```python
from build123d import *

# Parameters (mm, degrees)
SKETCH1_W                        = 20
SKETCH1_H                        = 20
BOSS_EXTRUDE1_DEPTH              = 30
F_3_0MM_DOWEL_HOLE1_D            = 3
F_3_0MM_DOWEL_HOLE1_DEPTH        = 20
F_3_0MM_DOWEL_HOLE1_CSINK_D      = 3.05
F_3_0MM_DOWEL_HOLE1_CSINK_ANGLE  = 90
F_3_0MM_DOWEL_HOLE1_TIP          = 0.901290929
F_3_0MM_DOWEL_HOLE2_D            = 3
F_3_0MM_DOWEL_HOLE2_DEPTH        = 12
F_3_0MM_DOWEL_HOLE2_CSINK_D      = 3.05
F_3_0MM_DOWEL_HOLE2_CSINK_ANGLE  = 90
F_3_0MM_DOWEL_HOLE2_TIP          = 0.901290929
F_3_0MM_DOWEL_HOLE3_D            = 3
F_3_0MM_DOWEL_HOLE3_DEPTH        = 20
F_3_0MM_DOWEL_HOLE3_CSINK_D      = 3.05
F_3_0MM_DOWEL_HOLE3_CSINK_ANGLE  = 90
F_3_0MM_DOWEL_HOLE3_TIP          = 0.901290929
F_10_0MM_DOWEL_HOLE1_D           = 9
F_10_0MM_DOWEL_HOLE1_DEPTH       = 17
F_10_0MM_DOWEL_HOLE1_CSINK_D     = 10.05
F_10_0MM_DOWEL_HOLE1_CSINK_ANGLE = 90
F_10_0MM_DOWEL_HOLE1_TIP         = 2.703872786


with BuildPart() as part:
    # Sketch1 → Boss-Extrude1 (new body)
    with BuildSketch(Plane(origin=(0, 0, 0), x_dir=(1, 0, 0), z_dir=(0, 1, 0))):
        with Locations((10, -8.099538279)):
            Rectangle(SKETCH1_W, SKETCH1_H)
    extrude(amount=BOSS_EXTRUDE1_DEPTH)

    # Ø3.0mm Dowel Hole1
    with Locations(Plane(origin=(0, 0, -1.900461721), x_dir=(-1, 0, 0), z_dir=(0, 0, -1))):
        with Locations((-16, 20)):
            CounterSinkHole(F_3_0MM_DOWEL_HOLE1_D / 2, F_3_0MM_DOWEL_HOLE1_CSINK_D / 2, depth=F_3_0MM_DOWEL_HOLE1_DEPTH, counter_sink_angle=F_3_0MM_DOWEL_HOLE1_CSINK_ANGLE)
            with Locations((0, 0, -(F_3_0MM_DOWEL_HOLE1_DEPTH + F_3_0MM_DOWEL_HOLE1_TIP / 2))):  # 118° drill point
                Cone(0, F_3_0MM_DOWEL_HOLE1_D / 2, F_3_0MM_DOWEL_HOLE1_TIP, mode=Mode.SUBTRACT)

    # Ø3.0mm Dowel Hole2
    with Locations(Plane.ZY):
        with Locations((10.099538279, 20)):
            CounterSinkHole(F_3_0MM_DOWEL_HOLE2_D / 2, F_3_0MM_DOWEL_HOLE2_CSINK_D / 2, depth=F_3_0MM_DOWEL_HOLE2_DEPTH, counter_sink_angle=F_3_0MM_DOWEL_HOLE2_CSINK_ANGLE)
            with Locations((0, 0, -(F_3_0MM_DOWEL_HOLE2_DEPTH + F_3_0MM_DOWEL_HOLE2_TIP / 2))):  # 118° drill point
                Cone(0, F_3_0MM_DOWEL_HOLE2_D / 2, F_3_0MM_DOWEL_HOLE2_TIP, mode=Mode.SUBTRACT)

    # Ø3.0mm Dowel Hole3
    with Locations(Plane(origin=(0, 30, 0), x_dir=(1, 0, 0), z_dir=(0, 1, 0))):
        with Locations((8, -4.099538279)):
            CounterSinkHole(F_3_0MM_DOWEL_HOLE3_D / 2, F_3_0MM_DOWEL_HOLE3_CSINK_D / 2, depth=F_3_0MM_DOWEL_HOLE3_DEPTH, counter_sink_angle=F_3_0MM_DOWEL_HOLE3_CSINK_ANGLE)
            with Locations((0, 0, -(F_3_0MM_DOWEL_HOLE3_DEPTH + F_3_0MM_DOWEL_HOLE3_TIP / 2))):  # 118° drill point
                Cone(0, F_3_0MM_DOWEL_HOLE3_D / 2, F_3_0MM_DOWEL_HOLE3_TIP, mode=Mode.SUBTRACT)

    # Ø10.0mm Dowel Hole1
    with Locations(Plane(origin=(20, 0, 0), x_dir=(0, 0, -1), z_dir=(1, 0, 0))):
        with Locations((-6.099538279, 8)):
            CounterSinkHole(F_10_0MM_DOWEL_HOLE1_D / 2, F_10_0MM_DOWEL_HOLE1_CSINK_D / 2, depth=F_10_0MM_DOWEL_HOLE1_DEPTH, counter_sink_angle=F_10_0MM_DOWEL_HOLE1_CSINK_ANGLE)
            with Locations((0, 0, -(F_10_0MM_DOWEL_HOLE1_DEPTH + F_10_0MM_DOWEL_HOLE1_TIP / 2))):  # 118° drill point
                Cone(0, F_10_0MM_DOWEL_HOLE1_D / 2, F_10_0MM_DOWEL_HOLE1_TIP, mode=Mode.SUBTRACT)


solid = part.part
```
The listing builds one solid part. Answer for the finished solid, in the listing's coordinates (mm). A direction names the side the tool comes from. Round coordinates to 2 decimals unless told otherwise and drop trailing zeros. Write each loop counter-clockwise with the first axis right and the second up, starting at its lowest first coordinate (ties: lowest second). Pieces come first, ordered by that corner, then holes. Notation, with made-up numbers: (11.5, -38) -> (38.5, -38) arc R19 ccw to (38.5, -27) -> close; hole circle Ø3 at (26, 64). An arc over 180 degrees is marked (long way). Use CSV: the item, a comma, the result in double quotes. Start each with the question number.
(1) Section B-B on x = 13.5 is taken. Give the vertices of the cut face in (y, z).
(2) The mould has two halves that part along Z. Classify faces 5 (the face through (14.89, 21.01, 8.25)), 6 (the face through (0.766, 8.775, 6.201)), 7 (the face through (10, 15, -1.9)): released by +Z, released by -Z, zero draft, split by the parting line, or undercut.
(3) Section D-D on y = 25.75 is taken. Give the vertices of the cut face in (x, z), then the cut area to 3 significant figures.
(4) Section A-A on x = 16 is taken. Give the vertices of the cut face in (y, z) (3 decimals).
(5) Consider L1, parallel to Z at x = 8, y = 19.25; L2, parallel to Y at x = 11.25, z = 9.75; L3, parallel to X at y = 20, z = 4.75. Determine where each line is inside the solid, lowest interval first. Write a range as from..to.
(6) Section C-C on x = 10 is taken. Give the vertices of the cut face in (y, z).
(7) Which of the six approach directions +Z, -Z, +X, -X, +Y, -Y give full straight-line access (tool end or side, diameter ignored) to faces 1 (the face through (11.12, 6.28, 10.26)), 2 (the face through (8.195, 20.268, 2.612)), 3 (the face through (6.096, 21.265, 9.293)), 4 (the face through (20, 15, 8))?
A:
1,outline,"(0, -1.9) -> (30, -1.9) -> (30, 18.1) -> (0, 18.1) -> close; hole circle Ø9 at (8, 6.1)"
2,face 5,"zero draft"
2,face 6,"undercut"
2,face 7,"released by -Z"
3,outline,"(0, -1.9) -> (20, -1.9) -> (20, 18.1) -> (0, 18.1) -> close; hole circle Ø3 at (8, 4.1)"
3,area,"393 mm²"
4,outline,"(0, -1.9) -> (18.475, -1.9) -> (18.5, -1.875) -> (18.5, 18.1) -> (0, 18.1) -> close; (21.5, -1.875) -> (21.525, -1.9) -> (30, -1.9) -> (30, 18.1) -> (21.5, 18.1) -> close; hole circle Ø9 at (8, 6.1)"
5,L1,"z = -1.9..2.6, 5.6..8.8, 11.4..18.1"
5,L2,"y = 0..5.37, 10.63..18.54, 21.46..30"
5,L3,"x = 0..6.65, 9.35..14.5, 17.5..20"
6,outline,"(0, -1.9) -> (30, -1.9) -> (30, 18.1) -> (0, 18.1) -> close; hole circle Ø9 at (8, 6.1); hole circle Ø3 at (20, 10.1)"
7,face 1,"+X"
7,face 2,"+Y"
7,face 3,"-X"
7,face 4,"+Z, -Z, +X, +Y, -Y"
